Build history of the part. All positions in model axes, mm. Face numbers are marked on the shaded views. Coordinates: 2 decimals unless noted, no trailing zeros. Order: outer loops, then holes, each group sorted by start corner. A loop starts at its lowest first (then second) coordinate and runs counter-clockwise, first axis right, second up. Notation, with made-up numbers: (80.5, 5.5) - (90.5, 5.5) arc R19 ccw to (90.5, 23.5) - close; hole circle Ø10 at (6.5, -24). An arc over 180 degrees is marked (long way). Write each question's results on one line, items separated by ' | '. Start each with the question number.
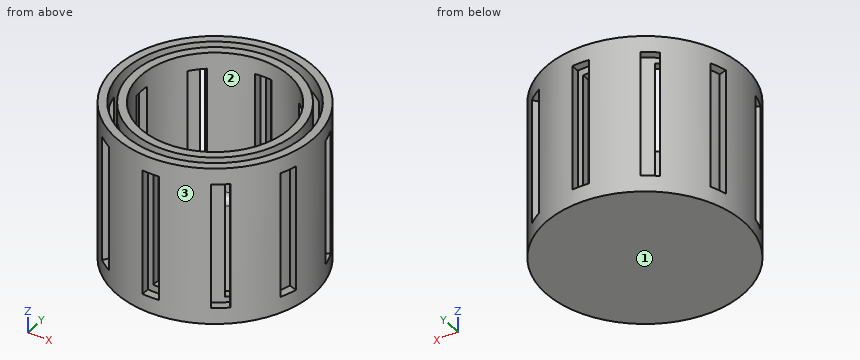
from build123d import *

# Parameters (mm, degrees)
F2_W            = 10
F2_H            = 76.3443418741
F3_REACH        = 136.997483921
F3_COPIES_COUNT = 8
F5_W            = 10
F5_H            = 76.3443418741
F6_REACH        = 211.997483921
F6_COPIES_COUNT = 10


# Not quite as in the source:
# - a pattern or mirror of a feature is missing from the dataset's text; its kind, count and spacing are read off the source's solid


with BuildPart() as f1:
    # F0 (on Front) → F1 (revolve)
    with BuildSketch(Plane.XZ):
        with BuildLine():
            Line((0, 5), (0, 0))
            Line((0, 0), (60, 0))
            Line((60, 0), (60, 96))
            Line((60, 96), (55, 96))
            Line((55, 96), (55, 5))
            Line((55, 5), (50, 5))
            Line((50, 5), (50, 96))
            Line((50, 96), (45, 96))
            Line((45, 96), (45, 10))
            ThreePointArc((45, 10), (43.5355339059, 6.4644660941), (40, 5))
            Line((40, 5), (0, 5))
        make_face()
    revolve(axis=Axis((0, 0, 2.5), (0, 0, 1)))

    f3_end = f1.faces().sort_by_distance((-50, 0, 50.5))[0]
    # F2 (on Front) → F3 (cut, up to a face of the model that its end follows)
    with BuildSketch(Plane.XZ):
        with Locations((0, 48)):
            Rectangle(F2_W, F2_H)
    f3_long = extrude(amount=F3_REACH, mode=Mode.PRIVATE)
    f3 = split(f3_long, bisect_by=f3_end, keep=Keep.BOTTOM, mode=Mode.PRIVATE)
    add(f3, mode=Mode.SUBTRACT)

    # F3_copies: F3 ×8 about axis
    f3_copies_axis = Axis((0, 0, 0), (0, 0, 1))
    for i in range(1, F3_COPIES_COUNT):
        add(f3.rotate(f3_copies_axis, i * 360 / F3_COPIES_COUNT), mode=Mode.SUBTRACT)

    f6_end = f1.faces().sort_by_distance((-55, 0, 50.5))[0]
    # F5 (on offset) → F6 (cut, up to a face of the model that its end follows)
    with BuildSketch(Plane.XZ.offset(75)):
        with Locations((0, 48)):
            Rectangle(F5_W, F5_H)
    f6_long = extrude(amount=-F6_REACH, mode=Mode.PRIVATE)
    f6 = split(f6_long, bisect_by=f6_end, keep=Keep.ALL, mode=Mode.PRIVATE).solids().sort_by_distance((0, -75, 48))[0]
    add(f6, mode=Mode.SUBTRACT)

    # F6_copies: F6 ×10 about axis
    f6_copies_axis = Axis((0, 0, 0), (0, 0, 1))
    for i in range(1, F6_COPIES_COUNT):
        add(f6.rotate(f6_copies_axis, i * 360 / F6_COPIES_COUNT), mode=Mode.SUBTRACT)


solid = f1.part
Item 1: Probe probe 1 along Y at (x, z) = (-0.5, 92); probe 2 along Y at (x, z) = (-41.5, 55); probe 3 along Z at (x, y) = (37, -32.5). List the from-to ranges inside material, lowest first.
Item 2: Slice it at B-B (y = 0). Write the cut outline in (x, z), then the cut area to 3 significant figures.
Item 3: Flat gauge pins, fed straight in: P1, Ø6, axis at x = 10.5, z = 18, coming from the -Y side; P2, Ø1.5, axis at x = -46, z = 31.5, coming from the -Y side; P3, Ø2.5, axis at y = 56, z = 64, coming from the +X side. Where does each tip first touch, or does it go through?
Item 4: Slice it at A-A (x = 0). Count the separate pieces of the cut face and the enclosed holes in it, then the cut area to 3 significant figures.
Item 5: Pull direction X, two halves, no side cores. Call the marked faces 1, 2 and 3: released by +X, released by -X, zero draft, split by the parting line, or undercut.
Resolved:
1) probe 1: -60 to -55, -50 to -45, 45 to 50, 55 to 60 | probe 2: -43.33 to -36.09, -27.89 to -17.4, 17.4 to 27.89, 36.09 to 43.33 | probe 3: 0 to 9.83, 86.17 to 96
2) outline: (-60, 0) - (60, 0) - (60, 96) - (55, 96) - (55, 5) - (50, 5) - (50, 9.83) - (45, 9.83) arc R5 cw to (40, 5) - (-40, 5) arc R5 cw to (-45, 9.83) - (-50, 9.83) - (-50, 5) - (-55, 5) - (-55, 96) - (-60, 96) - close; (-50, 86.17) - (-45, 86.17) - (-45, 96) - (-50, 96) - close; (45, 86.17) - (50, 86.17) - (50, 96) - (45, 96) - close | area: 1,670 mm^2
3) P1: y = -59.53 | P2: y = -39.4 | P3: x = 24.54
4) separate pieces: 5 | enclosed holes: 0 | area: 904 mm^2
5) face 1: zero draft | face 2: undercut | face 3: split by the parting line
